Verification items for this drawing (mm, ordinates from the low corner). Coordinates: 2 decimals unless noted, no trailing zeros. Order: outer loops, then holes, each group sorted by start corner. A loop starts at its lowest first (then second) coordinate and runs counter-clockwise, first axis right, second up. Notation, with made-up numbers: (74, -5) -> (80, -5) arc R13 ccw to (80, 3) -> close; hole circle Ø2 at (63, -14). An arc over 180 degrees is marked (long way). Write each question's results on one line, items separated by ' | '. Start each with the question number.
(1) Cross-section at A-A on y = 15. Enter the section's corners in (x, z), and give its area (3 significant figures).
(2) Cross-section at C-C on x = 175. Enter the section's corners in (y, z).
(3) Thickness scan on probe 1 along Y at (x, z) = (50, 7.25); probe 2 along Y at (x, z) = (150, 0.75); probe 3 along Y at (x, z) = (175, 3.5). Record the ranges inside material, lowest first. Write a range as [from, to].
(4) Cross-section at B-B on x = 150. Enter the section's corners in (y, z).
(5) Go/stop test with a flat-tipped pin: pin 1 (11 mm diameter, centred on x = 150, y = 45, fed in from +Z). Record where the tip stops, or that it passes through.
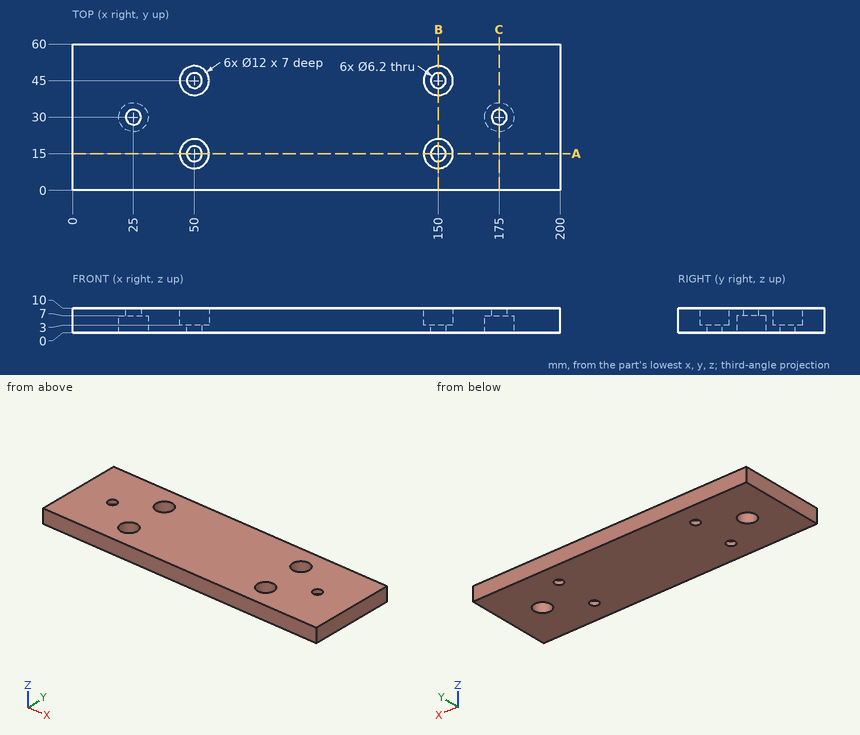
Results are:
1) outline: (0, 0) -> (46.9, 0) -> (46.9, 3) -> (44, 3) -> (44, 10) -> (0, 10) -> close; (53.1, 0) -> (146.9, 0) -> (146.9, 3) -> (144, 3) -> (144, 10) -> (56, 10) -> (56, 3) -> (53.1, 3) -> close; (153.1, 0) -> (200, 0) -> (200, 10) -> (156, 10) -> (156, 3) -> (153.1, 3) -> close | area: 1,790 mm2
2) outline: (0, 0) -> (24, 0) -> (24, 7) -> (26.9, 7) -> (26.9, 10) -> (0, 10) -> close; (33.1, 7) -> (36, 7) -> (36, 0) -> (60, 0) -> (60, 10) -> (33.1, 10) -> close
3) probe 1: y = [0, 9], [21, 39], [51, 60] | probe 2: y = [0, 11.9], [18.1, 41.9], [48.1, 60] | probe 3: y = [0, 24], [36, 60]
4) outline: (0, 0) -> (11.9, 0) -> (11.9, 3) -> (9, 3) -> (9, 10) -> (0, 10) -> close; (18.1, 0) -> (41.9, 0) -> (41.9, 3) -> (39, 3) -> (39, 10) -> (21, 10) -> (21, 3) -> (18.1, 3) -> close; (48.1, 0) -> (60, 0) -> (60, 10) -> (51, 10) -> (51, 3) -> (48.1, 3) -> close
5) pin 1: stops at z = 3
